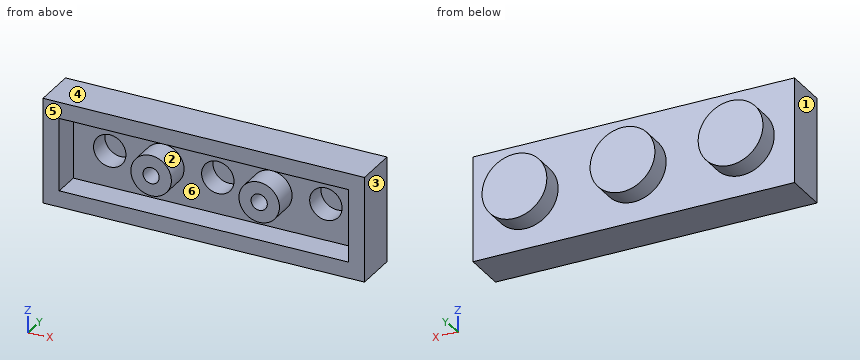
from build123d import *

# Parameters (mm, degrees)
SKETCH1_W            = 23.8
SKETCH1_H            = 3.2
BOSS_EXTRUDE1_DEPTH  = 7.8
SKETCH2_R            = 2.4
BOSS_EXTRUDE2_DEPTH  = 1.6
LPATTERN1_COUNT      = 2
LPATTERN1_PITCH      = 8
LPATTERN1_COUNT_DIR2 = 4
LPATTERN1_PITCH_DIR2 = 8
SHELL1_T             = -1.2
SKETCH3_R            = 1.5
SKETCH3_R_2          = 0.6
BOSS_EXTRUDE3_DEPTH  = 1.8
LPATTERN2_COUNT      = 2
LPATTERN2_PITCH      = 8


with BuildPart() as part:
    # Sketch1 → Boss-Extrude1 (new body)
    with BuildSketch(Plane.XY):
        with Locations((11.9, 1.6)):
            Rectangle(SKETCH1_W, SKETCH1_H)
    extrude(amount=-BOSS_EXTRUDE1_DEPTH)

    # Sketch2 → Boss-Extrude2 (add)
    with BuildSketch(Plane(origin=(0, 3.2, 0), x_dir=(1, 0, 0), z_dir=(0, 1, 0))):
        with Locations(Location((3.9, 3.9, 0), (0, 0, 270))):
            Circle(SKETCH2_R)
    boss_extrude2 = extrude(amount=BOSS_EXTRUDE2_DEPTH)

    # LPattern1: Boss-Extrude2 2 × 4, 5 skipped
    with Locations(*[(j * LPATTERN1_PITCH_DIR2, 0, i * LPATTERN1_PITCH) for i in range(LPATTERN1_COUNT) for j in range(LPATTERN1_COUNT_DIR2) if (i, j) not in ((0, 0), (0, 3), (1, 0), (1, 1), (1, 2), (1, 3))]):
        add(boss_extrude2)

    # Shell1
    shell1_openings = [part.faces().sort_by_distance(p)[0] for p in [
        (11.9, 0, -3.9),
    ]]
    offset(amount=SHELL1_T, openings=shell1_openings, kind=Kind.INTERSECTION)

    # Sketch3 → Boss-Extrude3 (add)
    with BuildSketch(Plane.XZ.offset(-2)):
        with Locations(Location((7.9, -3.9, 0), (0, 0, 90))):
            Circle(SKETCH3_R)
        with Locations(Location((7.9, -3.9, 0), (0, 0, 270))):
            Circle(SKETCH3_R_2, mode=Mode.SUBTRACT)
    boss_extrude3 = extrude(amount=BOSS_EXTRUDE3_DEPTH)

    # LPattern2: Boss-Extrude3 ×2
    with Locations(*[(i * LPATTERN2_PITCH, 0, 0) for i in range(1, LPATTERN2_COUNT)]):
        add(boss_extrude3)


solid = part.part
Design review of the part built by this model. Coordinates are the model's own, in mm. Face numbers are marked on the shaded views. A direction names the side the tool comes from. Coordinates: 2 decimals unless noted, no trailing zeros. Write each loop counter-clockwise with the first axis right and the second up, starting at its lowest first coordinate (ties: lowest second). Pieces come first, ordered by that corner, then holes. Notation, with made-up numbers: (27, -3.5) - (54, -3.5) arc R28 cw to (54, 18.5) - close; hole circle Ø4 at (-15, 81.25). An arc over 180 degrees is marked (long way). Use one line per item in the form item = value.
Q1. Consider section B-B (x = 7.9). Write out the cut boundary in (y, z).
Taken from the geometry:
outline = (0, -7.8) - (3.2, -7.8) - (3.2, 0) - (0, 0) - (0, -1.2) - (2, -1.2) - (2, -2.4) - (0.2, -2.4) - (0.2, -3.3) - (2, -3.3) - (2, -4.5) - (0.2, -4.5) - (0.2, -5.4) - (2, -5.4) - (2, -6.6) - (0, -6.6) - close
Q2. Consider section D-D (z = -2). Write out the cut boundary in (x, y), plus the area to 3 significant figures.
Taken from the geometry:
outline = (0, 0) - (1.2, 0) - (1.2, 2) - (22.6, 2) - (22.6, 0) - (23.8, 0) - (23.8, 3.2) - (21.37, 3.2) - (21.37, 4.8) - (18.43, 4.8) - (18.43, 3.2) - (13.37, 3.2) - (13.37, 4.8) - (10.43, 4.8) - (10.43, 3.2) - (5.37, 3.2) - (5.37, 4.8) - (2.43, 4.8) - (2.43, 3.2) - (0, 3.2) - close
area = 47.4 mm^2
Q3. The part is to be moulded in two halves that separate along X. For the marked faces 1, 2, 3 and 4, say which applies: +X half, -X half, draft (parallel to the pull), parting line (faces both ways), or undercut.
Taken from the geometry:
face_1 = -X half
face_2 = undercut
face_3 = +X half
face_4 = draft
Q4. Consider section C-C (y = 4.05). Write out the cut boundary in (x, z).
Taken from the geometry:
outline = circle Ø4.8 at (3.9, -3.9); circle Ø4.8 at (11.9, -3.9); circle Ø4.8 at (19.9, -3.9)
Q5. Machinability: for the marked faces 5 and 6, which of the approach directions +Z, -Z, +X, -X, +Y, -Y give a long, thin tool a straight path to every point of the face, cutting with its end or side? Answer none if there is none.
Taken from the geometry:
face_5 = +Z, -Z, +X, -X, -Y
face_6 = -Y
Q6. For probe 1 along X at (y, z) = (0.8, -3.9); probe 2 along Z at (x, y) = (7, 1.65); probe 3 along Z at (x, y) = (3.9, 2.9), list the stretches that pass through material, from the lowest coordinate up.
Taken from the geometry:
probe_1 = 0 to 1.2, 6.4 to 7.3, 8.5 to 9.4, 14.4 to 15.3, 16.5 to 17.4, 22.6 to 23.8
probe_2 = -7.8 to -6.6, -5.1 to -2.7, -1.2 to 0
probe_3 = -7.8 to -5.1, -2.7 to 0
Q7. Consider section A-A (y = 0.5). Write out the cut boundary in (x, z).
Taken from the geometry:
outline = (0, -7.8) - (23.8, -7.8) - (23.8, 0) - (0, 0) - close; circle Ø3 at (7.9, -3.9); circle Ø3 at (15.9, -3.9); hole (1.2, -6.6) - (22.6, -6.6) - (22.6, -1.2) - (1.2, -1.2) - close; hole circle Ø1.2 at (7.9, -3.9); hole circle Ø1.2 at (15.9, -3.9)
Q8. Insertion check: pin 1 Ø1.9 at (x, z) = (19.5, -3.5) entering from -Y; pin 2 Ø2 at (x, y) = (18.5, 2.5) entering from +Z; pin 3 Ø1.4 at (x, z) = (7.9, -3.9) entering from +Y; pin 4 Ø1 at (x, z) = (16, -4) entering from -Y. Each pin has a flat end and moves straight along its axis. Give the tip position at first contact, or say it passes through.
Taken from the geometry:
pin_1 = 2
pin_2 = 0
pin_3 = 3.2
pin_4 = 0.2
